Here's how the part is built. I have some questions about the finished solid (model axes, mm). A direction names the side the tool comes from. Coordinates: 2 decimals unless noted, no trailing zeros. Write each loop counter-clockwise with the first axis right and the second up, starting at its lowest first coordinate (ties: lowest second). Pieces come first, ordered by that corner, then holes. Notation, with made-up numbers: (55, 11) -> (84, 11) arc R11 ccw to (84, 28) -> close; hole circle Ø5 at (-6.5, 67.25). An arc over 180 degrees is marked (long way). Put each result on its own line as item: value. Start each with the question number.
Item 1: I need wall thicknesses on line 1 (X direction, y = -10.1, z = 46.85); line 2 (Y direction, x = 10.5, z = -1.9); line 3 (X direction, y = -10, z = -4). Which ranges of each line are inside material? Lowest first, please. Write a range as [from, to].
Item 2: I want a section at B-B, the plane z = 20.5. List the corners of the cut face in (x, y) for me.
Item 3: I want a section at A-A, the plane x = 10.5. List the corners of the cut face in (y, z) for me, then the cut area to 3 significant figures.
Item 4: I want a section at D-D, the plane z = 29. List the corners of the cut face in (x, y) for me.
Item 5: For pin 1 (0.8 mm diameter, centred on x = -17.5, y = -54, fed in from -Z); pin 2 (4 mm diameter, centred on x = 9.5, z = 7, fed in from -Y); pin 3 (6 mm diameter, centred on y = -28, z = 44, fed in from +X), each with a flat end and sliding along its axis, tell me the tip position at first contact or that it passes through.
Item 6: On a 3-axis mill with a long thin cutter (end or side, diameter ignored), from which of +Z, -Z, +X, -X, +Y, -Y can I reach the whole of each face in a straight line? I mean faces 5 (the face through (0, -23, -1)), 6 (the face through (-17, -55, 25.75)), 7 (the face through (21, -23, -1)), 8 (the face through (4.843, -9.943, 49.232)). Say none if no direction works.
Item 7: If we mould it in two halves opening along Y, with no side actions, what happens to faces 1 (the face through (-17.233, -61.057, 27.157)), 2 (the face through (9, -38, 23)), 3 (the face through (15.119, -12.015, 46.732)), 4 (the face through (6, -19, 50.5))? For each: released by +Y, released by -Y, zero draft, split by the parting line, or undercut.
Item 8: I want a section at C-C, the plane y = -10.1. List the corners of the cut face in (x, z) for me, then the cut area to 3 significant figures.
from build123d import *

# Parameters (mm, degrees)
CYLINDER039_R          = 3.4
CYLINDER039_DEPTH      = 44
CYLINDER038_R          = 5
CYLINDER038_DEPTH      = 9
PAD015_DEPTH           = 5
PAD014_DEPTH           = 21
CUT021_PITCH_ANGLE     = 90
CUT021_PLACEMENT_ANGLE = -180
CYLINDER037_R          = 3.4
CYLINDER037_DEPTH      = 44
CYLINDER036_R          = 5
CYLINDER036_DEPTH      = 9
PAD013_DEPTH           = 5
PAD012_DEPTH           = 21


with BuildPart() as cylinder039:
    # Cylinder039 → Cylinder039 (new body)
    with BuildSketch(Plane(origin=(10.5, -10.1, -9), x_dir=(1, 0, 0), z_dir=(0, 0, 1))):
        Circle(CYLINDER039_R)
    extrude(amount=CYLINDER039_DEPTH)


with BuildPart() as cylinder038:
    # Cylinder038 → Cylinder038 (new body)
    with BuildSketch(Plane(origin=(10.5, -10.1, 44), x_dir=(1, 0, 0), z_dir=(0, 0, 1))):
        Circle(CYLINDER038_R)
    extrude(amount=CYLINDER038_DEPTH)


with BuildPart() as fusion031:
    # Sketch015 → Pad015 (new body)
    with BuildSketch(Plane.XY):
        with BuildLine():
            Line((-4.25, 3.75), (-4.25, 9.25))
            Line((-4.25, 9.25), (-2.65, 17.292388))
            ThreePointArc((2.65, 17.292388), (0, 20), (-2.65, 17.292388))
            Line((2.65, 17.292388), (4.25, 9.25))
            Line((4.25, 3.75), (4.25, 9.25))
            ThreePointArc((4.25, -3.75), (5.657274, 0), (4.25, 3.75))
            Line((4.25, -3.75), (4.25, -9.25))
            Line((2.65, -17.292388), (4.25, -9.25))
            ThreePointArc((-2.65, -17.292388), (0, -20), (2.65, -17.292388))
            Line((-4.25, -9.25), (-2.65, -17.292388))
            Line((-4.25, -3.75), (-4.25, -9.25))
            ThreePointArc((-4.25, 3.75), (-5.657274, 0), (-4.25, -3.75))
        make_face()
    extrude(amount=PAD015_DEPTH)


with BuildPart() as fusion031_1:
    # Body015 placement: moved
    add(fusion031.part.moved(Location((10.5, -10, 48))))

    # Fusion031: union Cylinder038
    add(cylinder038.part)


with BuildPart() as obj1:
    # Sketch014 → Pad014 (new body)
    with BuildSketch(Plane.YZ):
        Polygon((-33, -0.5), (0, -0.5), (0, -5.5), (-38, -5.5), (-38, 50.5), (0, 50.5), (0, 45.5), (-33, 45.5), align=None)
    extrude(amount=PAD014_DEPTH)

    # Cut020: cut Fusion031
    add(fusion031_1.part, mode=Mode.SUBTRACT)

    # Cut021: cut Cylinder039
    add(cylinder039.part, mode=Mode.SUBTRACT)


with BuildPart() as obj1_1:
    # Cut021 pitch: moved
    add(obj1.part.rotate(Axis((0, 0, 0), (0, 1, 0)), CUT021_PITCH_ANGLE))


with BuildPart() as obj1_2:
    # Cut021 placement: moved
    add(obj1_1.part.moved(Location((32, -71, 32))).rotate(Axis((32, -71, 32), (0, 0, 1)), CUT021_PLACEMENT_ANGLE))


with BuildPart() as cylinder037:
    # Cylinder037 → Cylinder037 (new body)
    with BuildSketch(Plane(origin=(10.5, -10.1, -9), x_dir=(1, 0, 0), z_dir=(0, 0, 1))):
        Circle(CYLINDER037_R)
    extrude(amount=CYLINDER037_DEPTH)


with BuildPart() as cylinder036:
    # Cylinder036 → Cylinder036 (new body)
    with BuildSketch(Plane(origin=(10.5, -10.1, 44), x_dir=(1, 0, 0), z_dir=(0, 0, 1))):
        Circle(CYLINDER036_R)
    extrude(amount=CYLINDER036_DEPTH)


with BuildPart() as fusion030:
    # Sketch013 → Pad013 (new body)
    with BuildSketch(Plane.XY):
        with BuildLine():
            Line((-4.25, 3.75), (-4.25, 9.25))
            Line((-4.25, 9.25), (-2.65, 17.292388))
            ThreePointArc((2.65, 17.292388), (0, 20), (-2.65, 17.292388))
            Line((2.65, 17.292388), (4.25, 9.25))
            Line((4.25, 3.75), (4.25, 9.25))
            ThreePointArc((4.25, -3.75), (5.657274, 0), (4.25, 3.75))
            Line((4.25, -3.75), (4.25, -9.25))
            Line((2.65, -17.292388), (4.25, -9.25))
            ThreePointArc((-2.65, -17.292388), (0, -20), (2.65, -17.292388))
            Line((-4.25, -9.25), (-2.65, -17.292388))
            Line((-4.25, -3.75), (-4.25, -9.25))
            ThreePointArc((-4.25, 3.75), (-5.657274, 0), (-4.25, -3.75))
        make_face()
    extrude(amount=PAD013_DEPTH)


with BuildPart() as fusion030_1:
    # Body013 placement: moved
    add(fusion030.part.moved(Location((10.5, -10, 48))))

    # Fusion030: union Cylinder036
    add(cylinder036.part)


with BuildPart() as cadera:
    # Sketch012 → Pad012 (new body)
    with BuildSketch(Plane.YZ):
        Polygon((-33, -0.5), (0, -0.5), (0, -5.5), (-38, -5.5), (-38, 50.5), (0, 50.5), (0, 45.5), (-33, 45.5), align=None)
    extrude(amount=PAD012_DEPTH)

    # Cut018: cut Fusion030
    add(fusion030_1.part, mode=Mode.SUBTRACT)

    # Cut019: cut Cylinder037
    add(cylinder037.part, mode=Mode.SUBTRACT)

    # Fusion032: union obj1
    add(obj1_2.part)


solid = cadera.part
Calculated:
1. line 1: x = [0, 5.5], [15.5, 21]
1. line 2: y = [-38, -13.5], [-6.7, 0]
1. line 3: x = [0, 7.1], [13.9, 21]
2. outline: (-18.5, -41.2) -> (-16, -41.2) -> (-16, -56) -> (-13.5, -56) -> (-13.5, -38) -> (32.5, -38) -> (32.5, -57.65) -> (37.5, -57.65) -> (37.5, -33) -> (-18.5, -33) -> close; (-16, -71) -> (-13.5, -71) -> (-13.5, -65.8) -> (-16, -65.8) -> close; (32.5, -71) -> (37.5, -71) -> (37.5, -64.15) -> (32.5, -64.15) -> close
3. outline: (-38, -5.5) -> (-13.5, -5.5) -> (-13.5, -0.5) -> (-33, -0.5) -> (-33, 45.5) -> (-15.1, 45.5) -> (-15.1, 48) -> (-30, 48) -> (-30, 50.5) -> (-38, 50.5) -> close; (-6.7, -5.5) -> (0, -5.5) -> (0, -0.5) -> (-6.7, -0.5) -> close; (-5.1, 45.5) -> (0, 45.5) -> (0, 48) -> (-5.1, 48) -> close
3. area: 476 mm2
4. outline: (-18.5, -71) -> (-13.5, -71) -> (-13.5, -38) -> (32.5, -38) -> (32.5, -71) -> (37.5, -71) -> (37.5, -33) -> (-18.5, -33) -> close
5. pin 1: stops at z = 11
5. pin 2: stops at y = -38
5. pin 3: stops at x = 21
6. face 5: -Z, -X, +Y, -Y
6. face 6: -X
6. face 7: -Z, +X, +Y, -Y
6. face 8: +Z
7. face 1: undercut
7. face 2: released by -Y
7. face 3: undercut
7. face 4: zero draft
8. outline: (0, -5.5) -> (7.1, -5.5) -> (7.1, -0.5) -> (0, -0.5) -> close; (0, 45.5) -> (5.5, 45.5) -> (5.5, 48) -> (4.84, 48) -> (4.84, 50.5) -> (0, 50.5) -> close; (13.9, -5.5) -> (21, -5.5) -> (21, -0.5) -> (13.9, -0.5) -> close; (15.5, 45.5) -> (21, 45.5) -> (21, 50.5) -> (16.16, 50.5) -> (16.16, 48) -> (15.5, 48) -> close
8. area: 123 mm2
